Can you work these out from the model? Positions are in its coordinate system, mm. Coordinates: 2 decimals unless noted, no trailing zeros. Write each loop counter-clockwise with the first axis right and the second up, starting at its lowest first coordinate (ties: lowest second). Pieces come first, ordered by that corner, then holes. Notation, with made-up numbers: (41, 62) -> (73, 62) arc R16 ccw to (73, 77) -> close; hole circle Ø6 at (-15.75, 68.5). An arc over 180 degrees is marked (long way). Use one line per item in the form item = value.
```python
from build123d import *

# Parameters (mm, degrees)
SKETCH2_W           = 7.6
SKETCH2_H           = 7.6
BOSS_EXTRUDE1_DEPTH = 7.6
FILLET1_R           = 0.5
SKETCH3_R           = 1
CUT_EXTRUDE1_DEPTH  = 10
CUT_EXTRUDE2_REACH  = 13.4
SKETCH4_R           = 1


with BuildPart() as part:
    # Sketch2 → Boss-Extrude1 (new body)
    with BuildSketch(Plane(origin=(0, 0, 0), x_dir=(1, 0, 0), z_dir=(0, 1, 0))):
        Rectangle(SKETCH2_W, SKETCH2_H)
    extrude(amount=BOSS_EXTRUDE1_DEPTH)

    # Fillet1
    fillet1_edges = [part.edges().sort_by_distance(p)[0] for p in [
        (-3.8, 7.6, 0),
        (0, 7.6, 3.8),
        (3.8, 7.6, 0),
        (0, 0, 3.8),
        (-3.8, 0, 0),
        (0, 0, -3.8),
        (3.8, 0, 0),
        (3.8, 3.8, 3.8),
        (-3.8, 3.8, 3.8),
        (-3.8, 3.8, -3.8),
        (3.8, 3.8, -3.8),
        (0, 7.6, -3.8),
    ]]
    fillet(fillet1_edges, radius=FILLET1_R)

    # Sketch3 → Cut-Extrude1 (cut)
    with BuildSketch(Plane.ZY.offset(3.8)):
        with Locations((0, 3.8)):
            Circle(SKETCH3_R)
    extrude(amount=-CUT_EXTRUDE1_DEPTH, mode=Mode.SUBTRACT)

    # Cut-Extrude2: up to this face of the body (flat: up to its plane)
    cut_extrude2_end = Plane(part.part.faces().sort_by_distance((0, 3.8, -3.8))[0])
    # Sketch4 → Cut-Extrude2 (cut, up to the picked face)
    with BuildSketch(Plane.XY.offset(3.8), mode=Mode.PRIVATE) as cut_extrude2_sk1:
        with Locations((0, 3.8)):
            Circle(SKETCH4_R)
    cut_extrude2_tool1 = split(extrude(cut_extrude2_sk1.sketch, amount=-CUT_EXTRUDE2_REACH, mode=Mode.PRIVATE), bisect_by=cut_extrude2_end, keep=Keep.BOTH, mode=Mode.PRIVATE)
    add(cut_extrude2_tool1.solids().sort_by(Axis((0, 3.8, 3.8), (0, 0, -1)))[0], mode=Mode.SUBTRACT)


solid = part.part
```
Q1. Suppose I cut it at A-A (x = -2.5). Write out the boundary of the cut face in (y, z).
Return value:
outline = (0, -3.3) arc R0.5 ccw to (0.5, -3.8) -> (7.1, -3.8) arc R0.5 ccw to (7.6, -3.3) -> (7.6, 3.3) arc R0.5 ccw to (7.1, 3.8) -> (0.5, 3.8) arc R0.5 ccw to (0, 3.3) -> close; hole circle Ø2 at (3.8, 0)
Q2. If I drill on line 1 (X direction, y = 3.8, z = 2.15); line 2 (Y direction, x = 0, z = -2.2), over which ranges is the centre line in solid material (lowest first)? Write a range as from..to.
Return value:
line_1 = -3.8..-1, 1..3.8
line_2 = 0..2.8, 4.8..7.6
Q3. Will this pin go through, and if not, where does the flat tip stop? pin 1 (2.5 mm diameter, centred on x = 0, y = 3.8, fed in from -Z).
Return value:
pin_1 = -3.8
Q4. Suppose I cut it at B-B (y = 3.8). Write out the boundary of the cut face in (x, z), then the cut area to 3 significant figures.
Return value:
outline = (-3.8, -3.3) arc R0.5 ccw to (-3.3, -3.8) -> (-1, -3.8) -> (-1, -1) -> (-3.8, -1) -> close; (-3.8, 1) -> (-1, 1) -> (-1, 3.8) -> (-3.3, 3.8) arc R0.5 ccw to (-3.8, 3.3) -> close; (1, -3.8) -> (3.3, -3.8) arc R0.5 ccw to (3.8, -3.3) -> (3.8, -1) -> (1, -1) -> close; (1, 1) -> (3.8, 1) -> (3.8, 3.3) arc R0.5 ccw to (3.3, 3.8) -> (1, 3.8) -> close
area = 31.1 mm2
Q5. Thinking about a two-plate mould opening in Z: for faces 1 (the cylindrical face through (0.924, 3.417, 2.349)), 2 (the cylindrical face through (-2.349, 3.417, 0.924)), 3 (the flat face through (-1, 3, 3.8)), which applies, released by +Z, released by -Z, zero draft, split by the parting line, or undercut?
Return value:
face_1 = zero draft
face_2 = undercut
face_3 = released by +Z
Q6. Suppose I cut it at C-C (x = 0.5). Write out the boundary of the cut face in (y, z).
Return value:
outline = (0, -3.3) arc R0.5 ccw to (0.5, -3.8) -> (2.93, -3.8) -> (2.93, -0.5) arc R1 cw to (2.93, 0.5) -> (2.93, 3.8) -> (0.5, 3.8) arc R0.5 ccw to (0, 3.3) -> close; (4.67, -3.8) -> (7.1, -3.8) arc R0.5 ccw to (7.6, -3.3) -> (7.6, 3.3) arc R0.5 ccw to (7.1, 3.8) -> (4.67, 3.8) -> (4.67, 0.5) arc R1 cw to (4.67, -0.5) -> close
